Source: CAD feature listing. Evaluate the final solid. Frame: model axes, mm. Face numbers are marked on the shaded views. A direction names the side the tool comes from. Give positions to 0.01 mm unless a question says otherwise; leave off trailing zeros. Order: outer loops, then holes, each group sorted by start corner. A loop starts at its lowest first (then second) coordinate and runs counter-clockwise, first axis right, second up.
1) Section B-B, the plane y = -66. Return loops of the section in (x, z).
2) Access query for the marked faces 1 and 2. Directions: +Z, -Z, +X, -X, +Y, -Y. A direction counts if a zero-diameter tool reaches every point of the face in a straight line with its end or side. Return the directions, or none.
3) Section C-C, the plane z = 183.5. Return loops of the section in (x, y).
4) First-contact query: P1, Ø3, axis at x = -10, y = -58.5, coming from the -Z side; P2, Ø5, axis at x = 7.5, y = -64, coming from the -Z side; P3, Ø2, axis at x = -1.5, y = -49.5, coming from the +Z side. Flat tips, straight axial feed; report the tip coordinate or a pass-through.
5) Material intervals for line 1 (Y direction, x = 6, z = -37) (3 decimals); line 2 (Y direction, x = 10, z = 35); line 3 (Z direction, x = 13.5, y = -70), sorted ascending.
6) Section A-A, the plane x = 9. Return loops of the section in (y, z) (3 decimals).
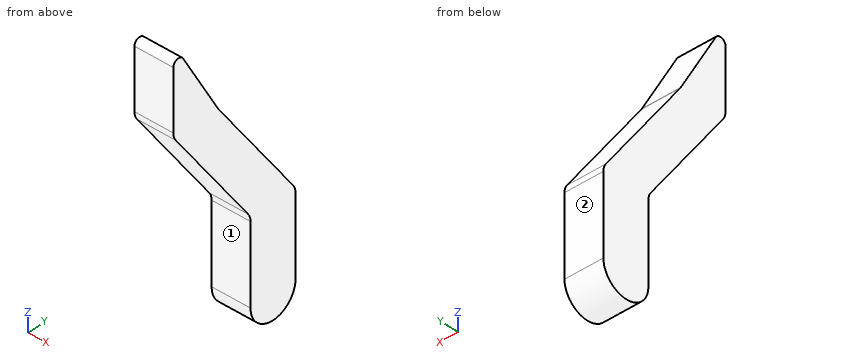
```python
from build123d import *

# Parameters (mm, degrees)
BOSS_EXTRUDE1_DEPTH = 17.78


with BuildPart() as part:
    # Sketch1 → Boss-Extrude1 (new body, symmetric)
    with BuildSketch(Plane(origin=(0, 0, 0), x_dir=(0, 0, -1), z_dir=(1, 0, 0))):
        with BuildLine():
            Line((-34.027638145, 22.225), (38.1, 22.225))
            ThreePointArc((38.1, 22.225), (60.325, 0), (38.1, -22.225))
            Line((38.1, -22.225), (-34.027638145, -22.225))
            ThreePointArc((-34.027638145, -22.225), (-37.905512075, -22.831526811), (-41.41298687, -24.593174207))
            Line((-41.41298687, -24.593174207), (-141.36658517, -96.041550766))
            ThreePointArc((-141.36658517, -96.041550766), (-144.874059965, -97.803198163), (-148.751933895, -98.409724974))
            Line((-148.751933895, -98.409724974), (-203.2806723, -98.409724974))
            ThreePointArc((-203.2806723, -98.409724974), (-208.190227055, -94.634589756), (-205.802839661, -88.920068321))
            Line((-205.802839661, -88.920068321), (-145.237041742, -54.278577891))
            ThreePointArc((-145.237041742, -54.278577891), (-144.688329899, -53.946063756), (-144.157111422, -53.586262051))
            Line((-144.157111422, -53.586262051), (-41.41298687, 19.856825793))
            ThreePointArc((-41.41298687, 19.856825793), (-37.905512075, 21.618473189), (-34.027638145, 22.225))
        make_face()
    extrude(amount=BOSS_EXTRUDE1_DEPTH, both=True)


solid = part.part
```
From the geometry:
1. outline: (-17.78, 99.34) - (17.78, 99.34) - (17.78, 165.73) - (-17.78, 165.73) - close
2. face 1: -Z, +X, -X, -Y
2. face 2: +Z, -Z, +X, -X, +Y
3. outline: (-17.78, -98.41) - (17.78, -98.41) - (17.78, -76.16) - (-17.78, -76.16) - close
4. P1: stops at z = 86.75
4. P2: stops at z = 93.04
4. P3: stops at z = 139.84
5. line 1: y = -22.225 to 22.225
5. line 2: y = -22.26 to 22.19
5. line 3: z = 104.94 to 172.72
6. outline: (-98.41, 148.752) arc R12.7 ccw to (-96.042, 141.367) - (-24.593, 41.413) arc R12.7 cw to (-22.225, 34.028) - (-22.225, -38.1) arc R22.225 ccw to (22.225, -38.1) - (22.225, 34.028) arc R12.7 ccw to (19.857, 41.413) - (-53.586, 144.157) arc R12.7 cw to (-54.279, 145.237) - (-88.92, 205.803) arc R5.08 ccw to (-98.41, 203.281) - close
